Can you work these out from the model? Positions are in its coordinate system, mm. Round coordinates to 2 decimals unless told otherwise and drop trailing zeros. Loops run counter-clockwise (first coordinate to the right, second up) from the corner with the lowest first, then second, coordinate; pieces in that order, holes last. Notation, with made-up numbers: M 52,-28.5 L 89,-28.5 A32 ccw 89,7.5 Z; hole C 24,19.25 d7. An arc over 180 degrees is marked long. Use a Markdown table: item, result. Add a question column.
```python
from build123d import *

# Parameters (mm, degrees)
F0_W      = 16.51
F0_H      = 16.51
F1_DEPTH  = 16.51
F2_SIZE   = 1.27
F3_W      = 4.064
F3_H      = 4.064
F4_DEPTH  = 5.08
F5_W      = 4.064
F5_H      = 4.064
F6_DEPTH  = 5.08
F7_W      = 4.064
F7_H      = 4.064
F8_DEPTH  = 5.08
F9_W      = 4.064
F9_H      = 4.064
F10_DEPTH = 5.08
F11_W     = 4.064
F11_H     = 4.064
F12_DEPTH = 5.08
F13_W     = 4.064
F13_H     = 4.064
F14_DEPTH = 5.08
F15_DEPTH = 1.016
F16_DEPTH = 1.016
F17_DEPTH = 1.016
F18_DEPTH = 1.016
F19_DEPTH = 1.016
F20_DEPTH = 1.016


with BuildPart() as f1:
    # F0 (on Top) → F1 (new body)
    with BuildSketch(Plane.XY):
        Rectangle(F0_W, F0_H)
    extrude(amount=F1_DEPTH)

    # F2
    f2_edges = [f1.edges().sort_by_distance(p)[0] for p in [
        (-8.255, 8.255, 8.255),
        (-8.255, -8.255, 8.255),
        (-8.255, 0, 0),
        (-8.255, 0, 16.51),
        (8.255, -8.255, 8.255),
        (0, -8.255, 16.51),
        (0, -8.255, 0),
        (8.255, 8.255, 8.255),
        (0, 8.255, 0),
        (0, 8.255, 16.51),
        (8.255, 0, 0),
        (8.255, 0, 16.51),
    ]]
    chamfer(f2_edges, length=F2_SIZE)

    # F3 (on face) → F4 (cut)
    with BuildSketch(Plane(origin=(0, 8.255, 0), x_dir=(-1, 0, 0), z_dir=(0, 1, 0))):
        with Locations((0, 8.255)):
            Rectangle(F3_W, F3_H)
    extrude(amount=-F4_DEPTH, mode=Mode.SUBTRACT)

    # F5 (on face) → F6 (cut)
    with BuildSketch(Plane.YZ.offset(8.255)):
        with Locations((0, 8.255)):
            Rectangle(F5_W, F5_H)
    extrude(amount=-F6_DEPTH, mode=Mode.SUBTRACT)

    # F7 (on face) → F8 (cut)
    with BuildSketch(Plane(origin=(-8.255, 0, 0), x_dir=(0, -1, 0), z_dir=(-1, 0, 0))):
        with Locations((0, 8.255)):
            Rectangle(F7_W, F7_H)
    extrude(amount=-F8_DEPTH, mode=Mode.SUBTRACT)

    # F9 (on face) → F10 (cut)
    with BuildSketch(Plane.XZ.offset(8.255)):
        with Locations((0, 8.255)):
            Rectangle(F9_W, F9_H)
    extrude(amount=-F10_DEPTH, mode=Mode.SUBTRACT)

    # F11 (on face) → F12 (cut)
    with BuildSketch(Plane.XY.offset(16.51)):
        Rectangle(F11_W, F11_H)
    extrude(amount=-F12_DEPTH, mode=Mode.SUBTRACT)

    # F13 (on face) → F14 (cut)
    with BuildSketch(Plane(origin=(0, 0, 0), x_dir=(1, 0, 0), z_dir=(0, 0, -1))):
        Rectangle(F13_W, F13_H)
    extrude(amount=-F14_DEPTH, mode=Mode.SUBTRACT)

    # F3 (on face) → F15 (join)
    with BuildSketch(Plane(origin=(0, 8.255, 0), x_dir=(-1, 0, 0), z_dir=(0, 1, 0))):
        with Locations((0, 8.255)):
            Rectangle(F3_W, F3_H)
    extrude(amount=-F15_DEPTH)

    # F5 (on face) → F16 (join)
    with BuildSketch(Plane.YZ.offset(8.255)):
        with Locations((0, 8.255)):
            Rectangle(F5_W, F5_H)
    extrude(amount=-F16_DEPTH)

    # F7 (on face) → F17 (join)
    with BuildSketch(Plane(origin=(-8.255, 0, 0), x_dir=(0, -1, 0), z_dir=(-1, 0, 0))):
        with Locations((0, 8.255)):
            Rectangle(F7_W, F7_H)
    extrude(amount=-F17_DEPTH)

    # F9 (on face) → F18 (join)
    with BuildSketch(Plane.XZ.offset(8.255)):
        with Locations((0, 8.255)):
            Rectangle(F9_W, F9_H)
    extrude(amount=-F18_DEPTH)

    # F11 (on face) → F19 (join)
    with BuildSketch(Plane.XY.offset(16.51)):
        Rectangle(F11_W, F11_H)
    extrude(amount=-F19_DEPTH)

    # F13 (on face) → F20 (join)
    with BuildSketch(Plane(origin=(0, 0, 0), x_dir=(1, 0, 0), z_dir=(0, 0, -1))):
        Rectangle(F13_W, F13_H)
    extrude(amount=-F20_DEPTH)


solid = f1.part
```
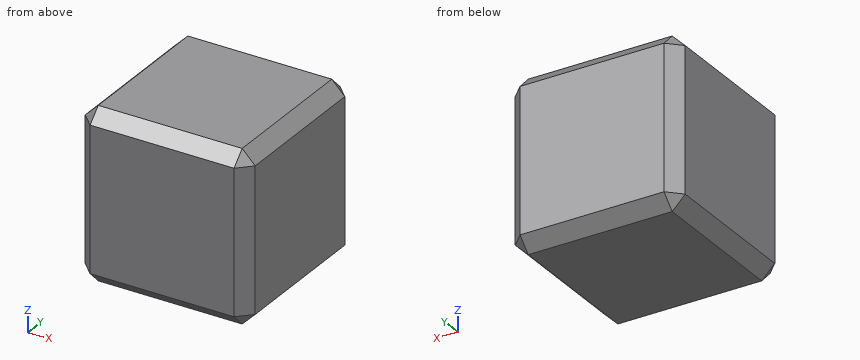
(1) If I drill on probe 1 along X at (y, z) = (-1.5, 8) (3 decimals); probe 2 along X at (y, z) = (0, 13) (3 decimals); probe 3 along Z at (x, y) = (6, -0.25), over which ranges is the centre line in solid material (lowest first)? Write a range as [from, to].
(2) Suppose I cut it at B-B on x = -1.5. List the corners of the cut face in (y, z) for me (3 decimals), and give its area (3 significant figures).
(3) Suppose I cut it at A-A on z = 9.5. List the corners of the cut face in (x, y) for me (3 decimals), and give its area (3 significant figures).
(4) Suppose I cut it at C-C on y = 4.25. List the corners of the cut face in (x, z) for me (3 decimals).
(5) Suppose I cut it at D-D on z = 14. List the corners of the cut face in (x, y) for me (3 decimals).
Results below:
| question | item | result |
|---|---|---|
| 1 | probe 1 | x = [-8.255, -7.239], [-3.175, 3.175], [7.239, 8.255] |
| 1 | probe 2 | x = [-8.255, -2.032], [2.032, 8.255] |
| 1 | probe 3 | z = [0, 6.22], [10.29, 16.51] |
| 2 | outline | M -8.255,1.27 L -6.985,0 L 6.985,0 L 8.255,1.27 L 8.255,15.24 L 6.985,16.51 L -6.985,16.51 L -8.255,15.24 Z; hole M -7.239,6.223 L -3.175,6.223 L -3.175,10.287 L -7.239,10.287 Z; hole M -2.032,1.016 L 2.032,1.016 L 2.032,5.08 L -2.032,5.08 Z; hole M -2.032,11.43 L 2.032,11.43 L 2.032,15.494 L -2.032,15.494 Z; hole M 3.175,6.223 L 7.239,6.223 L 7.239,10.287 L 3.175,10.287 Z |
| 2 | area | 203 mm² |
| 3 | outline | M -8.255,-6.985 L -6.985,-8.255 L 6.985,-8.255 L 8.255,-6.985 L 8.255,6.985 L 6.985,8.255 L -6.985,8.255 L -8.255,6.985 Z; hole M -7.239,-2.032 L -3.175,-2.032 L -3.175,2.032 L -7.239,2.032 Z; hole M -2.032,-7.239 L 2.032,-7.239 L 2.032,-3.175 L -2.032,-3.175 Z; hole M -2.032,3.175 L 2.032,3.175 L 2.032,7.239 L -2.032,7.239 Z; hole M 3.175,-2.032 L 7.239,-2.032 L 7.239,2.032 L 3.175,2.032 Z |
| 3 | area | 203 mm² |
| 4 | outline | M -8.255,1.27 L -6.985,0 L 6.985,0 L 8.255,1.27 L 8.255,15.24 L 6.985,16.51 L -6.985,16.51 L -8.255,15.24 Z; hole M -2.032,6.223 L 2.032,6.223 L 2.032,10.287 L -2.032,10.287 Z |
| 5 | outline | M -8.255,-6.985 L -6.985,-8.255 L 6.985,-8.255 L 8.255,-6.985 L 8.255,6.985 L 6.985,8.255 L -6.985,8.255 L -8.255,6.985 Z; hole M -2.032,-2.032 L 2.032,-2.032 L 2.032,2.032 L -2.032,2.032 Z |
